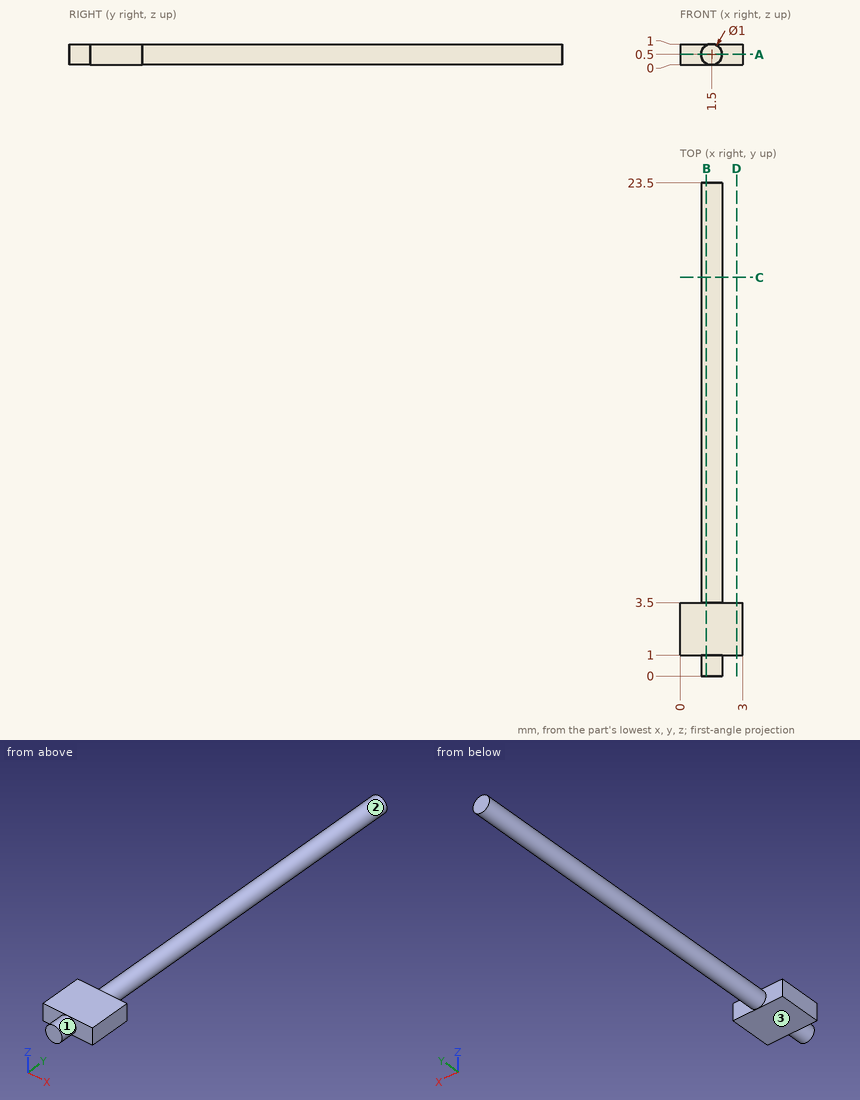
Verification items for this drawing (mm, ordinates from the low corner). A direction names the side the tool comes from. Round coordinates to 2 decimals unless told otherwise and drop trailing zeros. Order: outer loops, then holes, each group sorted by start corner. A loop starts at its lowest first (then second) coordinate and runs counter-clockwise, first axis right, second up. Notation, with made-up numbers: M 61.5,43.25 L 69.5,43.25 A27 ccw 69.5,59.25 Z; hole C 56.5,0.5 d7. An arc over 180 degrees is marked long. Answer in a Markdown table with one row per item. Add a question column.
Item 1: Material ranges on L1, parallel to Y at x = 2.05, z = 0.8; L2, parallel to X at y = 21.5, z = 0.5; L3, parallel to Z at x = 1.1, y = 16.25, recorded low to high. Write a range as [from, to].
Item 2: Set-up check for the marked faces 1, 2 and 3: record each of +Z, -Z, +X, -X, +Y, -Y from which the full face is reachable in a straight line by a thin tool's end or side.
Item 3: Sectioned sample at B-B, the plane x = 1.25. Enter the section's corners in (y, z), plus the area to 3 significant figures.
Item 4: Sectioned sample at A-A, the plane z = 0.5. Enter the section's corners in (x, y).
Item 5: Sectioned sample at C-C, the plane y = 19. Enter the section's corners in (x, z).
Item 6: Sectioned sample at D-D, the plane x = 2.7. Enter the section's corners in (y, z).
Filled in:
| question | item | result |
|---|---|---|
| 1 | L1 | y = [1, 3.5] |
| 1 | L2 | x = [1, 2] |
| 1 | L3 | z = [0.2, 0.8] |
| 2 | face 1 | -Y |
| 2 | face 2 | +Y |
| 2 | face 3 | -Z, +X, -X, +Y, -Y |
| 3 | outline | M 0,0.07 L 1,0.07 L 1,0 L 3.5,0 L 3.5,0.07 L 23.5,0.07 L 23.5,0.93 L 3.5,0.93 L 3.5,1 L 1,1 L 1,0.93 L 0,0.93 Z |
| 3 | area | 20.7 mm² |
| 4 | outline | M 0,1 L 1,1 L 1,0 L 2,0 L 2,1 L 3,1 L 3,3.5 L 2,3.5 L 2,23.5 L 1,23.5 L 1,3.5 L 0,3.5 Z |
| 5 | outline | C 1.5,0.5 d1 |
| 6 | outline | M 1,0 L 3.5,0 L 3.5,1 L 1,1 Z |
